from build123d import *

# Parameters (mm, degrees)
F0_R     = 11
F0_R_2   = 8.4
F1_DEPTH = 2.5
F0_R_3   = 6.35
F2_DEPTH = 35
F3_SIZE  = 0.6
F4_SIZE  = 1


with BuildPart() as f1:
    # F0 (on Right) → F1 (new body)
    with BuildSketch(Plane.YZ):
        Circle(F0_R)
        Circle(F0_R_2, mode=Mode.SUBTRACT)
    extrude(amount=F1_DEPTH)

    # F0 (on Right) → F2 (join)
    with BuildSketch(Plane.YZ):
        Circle(F0_R_2)
        Circle(F0_R_3, mode=Mode.SUBTRACT)
    extrude(amount=F2_DEPTH)

    # F3
    f3_edges = [f1.edges().sort_by_distance(p)[0] for p in [
        (35, -6.35, 0),
        (35, -8.4, 0),
        (0, -11, 0),
    ]]
    chamfer(f3_edges, length=F3_SIZE)

    # F4
    f4_edges = [f1.edges().sort_by_distance(p)[0] for p in [
        (0, -6.35, 0),
    ]]
    chamfer(f4_edges, length=F4_SIZE)


solid = f1.part
Read the model definition and answer for the solid it produces. Units are mm, in the model's axes. A direction names the side the tool comes from. Coordinates: 2 decimals unless noted, no trailing zeros. Loops run counter-clockwise (first coordinate to the right, second up) from the corner with the lowest first, then second, coordinate; pieces in that order, holes last. Notation, with made-up numbers: (-11.75, 43) -> (34.25, 43) arc R18 ccw to (34.25, 78) -> close; hole circle Ø6 at (31.5, 3). An arc over 180 degrees is marked (long way). Answer in a Markdown table with one row per item.
Item 1: Each of these flat-tipped pins is pushed along its axis until it touches: P1, Ø1, axis at x = 26.5, y = 6, coming from the -Z side; P2, Ø12, axis at x = 30, y = -3, coming from the +Z side; P3, Ø1, axis at x = 5.5, y = 5, coming from the +Z side; P4, Ø4, axis at y = 8, z = 3, coming from the -X side. Where does it stop, or does it pass through?
Returned:
| item | result |
|---|---|
| P1 | stops at z = -6.35 |
| P2 | stops at z = 8.4 |
| P3 | stops at z = 7.09 |
| P4 | stops at x = 0 |
Item 2: For a pull along Y with two mould halves and no side action, classify faces 1 (the cylindrical face through (17.47, -1.38, -6.2)), 2 (the cylindrical face through (1.54, -2.38, -10.74)), 3 (the flat face through (2.5, 3.2, -8.1)) as released by +Y, released by -Y, zero draft, split by the parting line, or undercut.
Returned:
| item | result |
|---|---|
| face 1 | undercut |
| face 2 | split by the parting line |
| face 3 | zero draft |
Item 3: A cutting plane is placed at C-C on x = 6.5. Determine the outline of the cut face in (y, z).
Returned:
| item | result |
|---|---|
| outline | circle Ø16.8 at (0, 0); hole circle Ø12.7 at (0, 0) |
Item 4: A cutting plane is placed at A-A on y = 0. Determine the outline of the cut face in (x, z).
Returned:
| item | result |
|---|---|
| outline | (0, -10.4) -> (0.6, -11) -> (2.5, -11) -> (2.5, -8.4) -> (34.4, -8.4) -> (35, -7.8) -> (35, -6.95) -> (34.4, -6.35) -> (1, -6.35) -> (0, -7.35) -> close; (0, 7.35) -> (1, 6.35) -> (34.4, 6.35) -> (35, 6.95) -> (35, 7.8) -> (34.4, 8.4) -> (2.5, 8.4) -> (2.5, 11) -> (0.6, 11) -> (0, 10.4) -> close |
Item 5: Straight lines are drawn through the part: line 1 along Z through (x, y) = (17.5, 0); line 2 along X through (y, z) = (-9.75, 3.25); line 3 along Y through (x, z) = (21.5, -2). For each, find the intervals that lie inside material, in ascending order. Write a range as [from, to].
Returned:
| item | result |
|---|---|
| line 1 | z = [-8.4, -6.35], [6.35, 8.4] |
| line 2 | x = [0, 2.5] |
| line 3 | y = [-8.16, -6.03], [6.03, 8.16] |
Item 6: For faces 4 (the cylindrical face through (18.227, 8.012, 2.523)), 5 (the flat face through (0, -2.5, 7.1)), determine the directions among +Z, -Z, +X, -X, +Y, -Y from which every point of the face is accessible in a straight line to the end or side of a thin tool.
Returned:
| item | result |
|---|---|
| face 4 | +X |
| face 5 | +Z, -Z, -X, +Y, -Y |
